Part model, mm, in its own coordinate system. A direction names the side the tool comes from. Coordinates: 2 decimals unless noted, no trailing zeros. Loops run counter-clockwise (first coordinate to the right, second up) from the corner with the lowest first, then second, coordinate; pieces in that order, holes last. Notation, with made-up numbers: (44, 53) -> (93, 53) arc R31 cw to (93, 89) -> close; hole circle Ø2 at (84, 1). An arc over 180 degrees is marked (long way). One line per question, with ' | ' between items. Start each with the question number.
1) 3-axis set-ups, long thin cutter, end or side, ignore diameter. For faces 1 (the face through (0, 5, -12.5)), 2 (the face through (21, 97, -37.5)), 3 (the face through (21, 3, -37.5)), 4 (the face through (-21, 51, 0)): which of +Z, -Z, +X, -X, +Y, -Y reach the whole face in a straight line?
2) Cut at A-A (z = -90). List the corners of the cut face in (x, y).
3) Cut at C-C (y = 50). List the corners of the cut face in (x, z).
4) Cut at D-D (y = 73.5). List the corners of the cut face in (x, z).
5) Cut at B-B (x = 0). List the corners of the cut face in (y, z).
6) Probe L1, parallel to X at y = 17, z = -68; L2, parallel to Y at x = -16, z = -12; L3, parallel to X at y = 55.5, z = -58.5. List the from-to ranges inside material, lowest first. Write a range as from..to.
7) Drop flat-ended pins along their axis: pin 1 (1.8 mm diameter, centred on x = 23, y = 97, fed in from +Z); pin 2 (2 mm diameter, centred on x = -28, z = -42, fed in from -Y); pin 3 (1 mm diameter, centred on x = -23.5, y = 49, fed in from -Z); pin 4 (1 mm diameter, centred on x = 13, y = 29, fed in from +Z). Give the stop position or say it passes through.
8) Two-plate mould, pull along X, no slides. Class faces 5 (the face through (-18.101, 5.577, 15.282)), 6 (the face through (-21, 94, -25)), 7 (the face through (0, 11, 4)): released by +X, released by -X, zero draft, split by the parting line, or undercut.
from build123d import *

# Parameters (mm, degrees)
BOSS_EXTRUDE1_START = 18
BOSS_EXTRUDE1_DEPTH = 7
BOSS_EXTRUDE3_START = -18
BOSS_EXTRUDE3_DEPTH = 7
BOSS_EXTRUDE4_DEPTH = 11
BOSS_EXTRUDE5_START = -11
BOSS_EXTRUDE5_DEPTH = 11
SKETCH9_R           = 12.5
BOSS_EXTRUDE6_DEPTH = 28
BOSS_EXTRUDE7_START = -28
SKETCH11_R          = 12.5
BOSS_EXTRUDE7_DEPTH = 28
HOLE1_D             = 18
SKETCH14_R          = 15
BOSS_EXTRUDE8_DEPTH = 12
HOLE2_D             = 14


with BuildPart() as part:
    # Sketch1 → Boss-Extrude1 (new body)
    with BuildSketch(Plane(origin=(0, 0, 0), x_dir=(0, 0, -1), z_dir=(1, 0, 0)).offset(BOSS_EXTRUDE1_START)):
        with BuildLine():
            Line((0, 0), (12.5, 0))
            Line((12.5, 0), (12.5, 6))
            Line((12.5, 6), (37.5, 6))
            Line((37.5, 6), (37.5, 0))
            Line((37.5, 0), (50, 0))
            ThreePointArc((50, 0), (100, 50), (50, 100))
            Line((50, 100), (37.5, 100))
            Line((37.5, 100), (37.5, 94))
            Line((37.5, 94), (12.5, 94))
            Line((12.5, 94), (12.5, 100))
            Line((12.5, 100), (0, 100))
            Line((0, 100), (0, 0))
        make_face()
    extrude(amount=BOSS_EXTRUDE1_DEPTH)



with BuildPart() as body_2:
    # Sketch3 → Boss-Extrude3 (new body)
    with BuildSketch(Plane(origin=(0, 0, 0), x_dir=(0, 0, -1), z_dir=(1, 0, 0)).offset(BOSS_EXTRUDE3_START)):
        with BuildLine():
            Line((0, 100), (0, 0))
            Line((0, 0), (12.5, 0))
            Line((12.5, 0), (12.5, 6))
            Line((12.5, 6), (37.5, 6))
            Line((37.5, 6), (37.5, 0))
            Line((37.5, 0), (50, 0))
            ThreePointArc((50, 0), (100, 50), (50, 100))
            Line((50, 100), (37.5, 100))
            Line((37.5, 100), (37.5, 94))
            Line((37.5, 94), (12.5, 94))
            Line((12.5, 94), (12.5, 100))
            Line((12.5, 100), (0, 100))
        make_face()
    extrude(amount=-BOSS_EXTRUDE3_DEPTH)


with BuildPart() as part_1:
    add(part.part)

    add(body_2.part)  # Boss-Extrude4 merges body 2
    # Sketch5 → Boss-Extrude4 (add)
    with BuildSketch(Plane(origin=(0, 100, 0), x_dir=(1, 0, 0), z_dir=(0, 1, 0))):
        with BuildLine():
            Line((-25, 12.5), (25, 12.5))
            Line((25, 12.5), (25, 0))
            Line((25, 0), (11.392973, -30.142973))
            ThreePointArc((11.392973, -30.142973), (0, -37.5), (-11.392973, -30.142973))
            Line((-11.392973, -30.142973), (-25, 0))
            Line((-25, 0), (-25, 12.5))
        make_face()
    extrude(amount=-BOSS_EXTRUDE4_DEPTH)

    # Sketch8 → Boss-Extrude5 (add)
    with BuildSketch(Plane.XZ.offset(BOSS_EXTRUDE5_START)):
        with BuildLine():
            Line((-25, 0), (-25, -12.5))
            Line((-25, -12.5), (-18, -12.5))
            Line((-18, -12.5), (18, -12.5))
            Line((18, -12.5), (25, -12.5))
            Line((25, -12.5), (25, 0))
            Line((25, 0), (11.392973, 30.142973))
            ThreePointArc((11.392973, 30.142973), (0, 37.5), (-11.392973, 30.142973))
            Line((-11.392973, 30.142973), (-25, 0))
        make_face()
    extrude(amount=BOSS_EXTRUDE5_DEPTH)

    # Sketch9 → Boss-Extrude6 (add)
    with BuildSketch(Plane(origin=(0, 100, 0), x_dir=(1, 0, 0), z_dir=(0, 1, 0))):
        with Locations(Location((0, -25, 0), (0, 0, 270))):
            Circle(SKETCH9_R)
    extrude(amount=-BOSS_EXTRUDE6_DEPTH)

    # Sketch11 → Boss-Extrude7 (add)
    with BuildSketch(Plane.XZ.offset(BOSS_EXTRUDE7_START)):
        with Locations(Location((0, 25, 0), (0, 0, 90))):
            Circle(SKETCH11_R)
    extrude(amount=BOSS_EXTRUDE7_DEPTH)

    # Hole1 (through all)
    with Locations(Plane(origin=(0, 0, 0), x_dir=(-1, 0, 0), z_dir=(0, -1, 0))):
        with Locations((0, -25)):
            Hole(HOLE1_D / 2)

    # Sketch14 → Boss-Extrude8 (add)
    with BuildSketch(Plane.ZY.offset(25)):
        with Locations((-50, 50)):
            Circle(SKETCH14_R)
    boss_extrude8 = extrude(amount=BOSS_EXTRUDE8_DEPTH)

    # Mirror1: Boss-Extrude8 across plane
    add(boss_extrude8.mirror(Plane(origin=(0, 0, 0), x_dir=(0, 0, 1), z_dir=(1, 0, 0))))

    # Hole2 (through all)
    with Locations(Plane(origin=(37, 0, 0), x_dir=(0, 0, -1), z_dir=(1, 0, 0))):
        with Locations((50, 50)):
            Hole(HOLE2_D / 2)


solid = part_1.part
Reported:
1) face 1: -Y | face 2: +X, -X, +Y | face 3: +X, -X, -Y | face 4: +Z, +X, -X
2) outline: (-25, 20) -> (-18, 20) -> (-18, 80) -> (-25, 80) -> close; (18, 20) -> (25, 20) -> (25, 80) -> (18, 80) -> close
3) outline: (-37, -65) -> (-25, -65) -> (-25, -100) -> (-18, -100) -> (-18, -57) -> (-37, -57) -> close; (-37, -43) -> (-18, -43) -> (-18, 0) -> (-25, 0) -> (-25, -35) -> (-37, -35) -> close; (18, -100) -> (25, -100) -> (25, -65) -> (37, -65) -> (37, -57) -> (18, -57) -> close; (18, -43) -> (37, -43) -> (37, -35) -> (25, -35) -> (25, 0) -> (18, 0) -> close
4) outline: (-25, -94.13) -> (-18, -94.13) -> (-18, 0) -> (-25, 0) -> close; circle Ø25 at (0, 25); (18, -94.13) -> (25, -94.13) -> (25, 0) -> (18, 0) -> close; hole circle Ø18 at (0, 25)
5) outline: (0, -12.5) -> (11, -12.5) -> (11, 12.5) -> (28, 12.5) -> (28, 16) -> (0, 16) -> close; (0, 34) -> (28, 34) -> (28, 37.5) -> (0, 37.5) -> close; (72, 12.5) -> (89, 12.5) -> (89, -12.5) -> (100, -12.5) -> (100, 16) -> (72, 16) -> close; (72, 34) -> (100, 34) -> (100, 37.5) -> (72, 37.5) -> close
6) L1: x = -25..-18, 18..25 | L2: y = 0..11, 89..100 | L3: x = -37..-18, 18..37
7) pin 1: stops at z = 6.42 | pin 2: stops at y = 36.73 | pin 3: stops at z = -100 | pin 4: passes through
8) face 5: released by -X | face 6: zero draft | face 7: undercut
